Could you check a few things on this model? Use its own coordinates, in mm. A direction names the side the tool comes from. Round coordinates to 2 decimals unless told otherwise and drop trailing zeros. Loops run counter-clockwise (first coordinate to the right, second up) from the corner with the lowest first, then second, coordinate; pieces in that order, holes last. Notation, with made-up numbers: (57, -21.75) -> (82, -21.75) arc R21 ccw to (82, 16.25) -> close; hole circle Ø3 at (25, 86). An arc over 180 degrees is marked (long way). One line per item, written item: value.
```python
from build123d import *

# Parameters (mm, degrees)
SKETCH1_R           = 2.5
BOSS_EXTRUDE3_DEPTH = 18.5
CUT_EXTRUDE2_START  = -9
CUT_EXTRUDE2_DEPTH  = 9
SKETCH1_5_W         = 7
SKETCH1_5_H         = 33
SKETCH1_5_R         = 2.5
SKETCH1_5_H_2       = 65
BOSS_EXTRUDE4_DEPTH = 18.825
SKETCH3_R           = 17.825
CUT_EXTRUDE3_DEPTH  = 176.104627652


with BuildPart() as part:
    # Sketch1 → Boss-Extrude3 (new body)
    with BuildSketch(Plane.XY):
        with BuildLine():
            Line((161.5, 32.5), (147, 32.5))
            Line((147, 32.5), (106.5, 32.5))
            Line((106.5, 32.5), (106.5, -32.5))
            Line((106.5, -32.5), (147, -32.5))
            Line((147, -32.5), (161.5, -32.5))
            Line((161.5, -32.5), (161.5, -10.25))
            Line((161.5, -10.25), (153, -10.25))
            ThreePointArc((153, -10.25), (148.757359313, -12.007359313), (147, -16.25))
            Line((147, -16.25), (147, -26))
            Line((147, -26), (114.5, -26))
            Line((114.5, -26), (114.5, 26))
            Line((114.5, 26), (147, 26))
            Line((147, 26), (147, 16.25))
            ThreePointArc((147, 16.25), (148.757359313, 12.007359313), (153, 10.25))
            Line((153, 10.25), (161.5, 10.25))
            Line((161.5, 10.25), (161.5, 32.5))
        make_face()
        with Locations((153, -16.25)):
            Circle(SKETCH1_R, mode=Mode.SUBTRACT)
        with Locations((153, 16.25)):
            Circle(SKETCH1_R, mode=Mode.SUBTRACT)
    extrude(amount=BOSS_EXTRUDE3_DEPTH)

    # Sketch2 → Cut-Extrude2 (cut)
    with BuildSketch(Plane.XY.offset(18.5).offset(CUT_EXTRUDE2_START)):
        with BuildLine():
            Line((153, 22.25), (147, 22.25))
            Line((147, 22.25), (147, 10.25))
            Line((147, 10.25), (159, 10.25))
            Line((159, 10.25), (159, 16.25))
            ThreePointArc((159, 16.25), (157.242640687, 20.492640687), (153, 22.25))
        make_face()
        with BuildLine():
            Line((153, -22.25), (147, -22.25))
            Line((147, -22.25), (147, -10.25))
            Line((147, -10.25), (159, -10.25))
            Line((159, -10.25), (159, -16.25))
            ThreePointArc((159, -16.25), (157.242640687, -20.492640687), (153, -22.25))
        make_face()
    extrude(amount=CUT_EXTRUDE2_DEPTH, mode=Mode.SUBTRACT)

    # Sketch1_5 → Boss-Extrude4 (add)
    # profile 1 of 3: a face of its own
    with BuildSketch(Plane.XY):
        with BuildLine():
            Line((99.5, -32.5), (99.5, 32.5))
            Line((99.5, 32.5), (62.5, 32.5))
            Line((62.5, 32.5), (62.5, -0.5))
            ThreePointArc((62.5, -0.5), (70.731609419, -15.568030239), (73.58, -32.5))
            Line((73.58, -32.5), (99.5, -32.5))
        make_face()
    # profile 2 of 3: a face of its own
    with BuildSketch(Plane.XY):
        with Locations((59, 16)):
            Rectangle(SKETCH1_5_W, SKETCH1_5_H)
        with Locations(Location((59, 7.5, 0), (0, 0, 180))):
            Circle(SKETCH1_5_R, mode=Mode.SUBTRACT)
        with Locations(Location((59, 24.5, 0), (0, 0, 180))):
            Circle(SKETCH1_5_R, mode=Mode.SUBTRACT)
    # profile 3 of 3: a face of its own
    with BuildSketch(Plane.XY):
        with Locations((103, 0)):
            Rectangle(SKETCH1_5_W, SKETCH1_5_H_2)
        with Locations(Location((103, -16.25, 0), (0, 0, 180))):
            Circle(SKETCH1_5_R, mode=Mode.SUBTRACT)
        with Locations(Location((103, 16.25, 0), (0, 0, 180))):
            Circle(SKETCH1_5_R, mode=Mode.SUBTRACT)
    extrude(amount=BOSS_EXTRUDE4_DEPTH)

    # Sketch3 → Cut-Extrude3 (cut, through all)
    with BuildSketch(Plane.XZ.offset(32.5)):
        with Locations((80.325, 18.825)):
            Circle(SKETCH3_R)
    extrude(amount=-CUT_EXTRUDE3_DEPTH, mode=Mode.SUBTRACT)


solid = part.part
```
(1) For pin 1 Ø4.5 at (x, y) = (103, 16.25) entering from +Z; pin 2 Ø5 at (x, y) = (115, 1.5) entering from +Z; pin 3 Ø6 at (x, y) = (153, -16.25) entering from +Z; pin 4 Ø3 at (y, z) = (-23.5, 9.5) entering from -X, each with a flat end and sliding along its axis, tell me the tip position at first contact or that it passes through.
Results below:
pin 1: passes through
pin 2: stops at z = 18.5
pin 3: stops at z = 9.5
pin 4: stops at x = 94.49
(2) Imagine slicing it at D-D on x = 59. Write out the boundary of the cut face in (y, z) (3 decimals).
Results below:
outline: (-0.5, 0) -> (5, 0) -> (5, 18.825) -> (-0.5, 18.825) -> close; (10, 0) -> (22, 0) -> (22, 18.825) -> (10, 18.825) -> close; (27, 0) -> (32.5, 0) -> (32.5, 18.825) -> (27, 18.825) -> close
(3) We'd pull the mould along Y, two halves only. Please class faces 1 (the face through (114.5, 0, 9)), 2 (the face through (68.239, -9.603, 3.791)), 3 (the face through (161.5, 21, 9)): +Y half, -Y half, draft (parallel to the pull), parting line (faces both ways), or undercut.
Results below:
face 1: undercut
face 2: -Y half
face 3: draft
(4) Imagine slicing it at C-C on z = 13.25. Write out the boundary of the cut face in (x, y), then the cut area to 3 significant figures.
Results below:
outline: (55.5, -0.5) -> (62.5, -0.5) arc R51.75 cw to (63.39, -1.67) -> (63.39, 32.5) -> (55.5, 32.5) -> close; (97.26, -32.5) -> (161.5, -32.5) -> (161.5, -10.25) -> (159, -10.25) -> (159, -16.25) arc R6 cw to (153, -22.25) -> (147, -22.25) -> (147, -26) -> (114.5, -26) -> (114.5, 26) -> (147, 26) -> (147, 22.25) -> (153, 22.25) arc R6 cw to (159, 16.25) -> (159, 10.25) -> (161.5, 10.25) -> (161.5, 32.5) -> (97.26, 32.5) -> close; hole circle Ø5 at (59, 7.5); hole circle Ø5 at (59, 24.5); hole circle Ø5 at (103, -16.25); hole circle Ø5 at (103, 16.25)
area: 2,100 mm²
(5) On a 3-axis mill with a long thin cutter (end or side, diameter ignored), from which of +Z, -Z, +X, -X, +Y, -Y can I reach the whole of each face in a straight line? I mean faces 4 (the face through (157.289, -20.446, 13.937)), 5 (the face through (55.5, 16, 9)), 6 (the face through (59, 16, 18.825)), 7 (the face through (59, -0.5, 9)), 8 (the face through (147, 22, 7)). Say none if no direction works.
Results below:
face 4: +Z
face 5: +Z, -Z, -X, +Y, -Y
face 6: +Z, +X, -X, +Y, -Y
face 7: +Z, -Z, -X, -Y
face 8: +Z, -Z
(6) Imagine slicing it at B-B on x = 128.5. Write out the boundary of the cut face in (y, z).
Results below:
outline: (-32.5, 0) -> (-26, 0) -> (-26, 18.5) -> (-32.5, 18.5) -> close; (26, 0) -> (32.5, 0) -> (32.5, 18.5) -> (26, 18.5) -> close
(7) Imagine slicing it at A-A on y = 7.5. Write out the boundary of the cut face in (x, z) (3 decimals).
Results below:
outline: (55.5, 0) -> (56.5, 0) -> (56.5, 18.825) -> (55.5, 18.825) -> close; (61.5, 0) -> (114.5, 0) -> (114.5, 18.5) -> (106.5, 18.5) -> (106.5, 18.825) -> (98.15, 18.825) arc R17.825 cw to (62.5, 18.825) -> (61.5, 18.825) -> close
(8) Please list where these lines run through material, in increasing order: L1, parallel to Y at x = 153, z = 2.75; L2, parallel to Y at x = 59, z = 8.25.
Results below:
L1: y = -32.5 to -18.75, -13.75 to -10.25, 10.25 to 13.75, 18.75 to 32.5
L2: y = -0.5 to 5, 10 to 22, 27 to 32.5
